```python
from build123d import *

# Parameters (mm, degrees)
EXTRUDE_1_DEPTH     = 1.5
HOLE_WIZARD_M4_1_D  = 4.2
HOLE_WIZARD_M8_1_D  = 8.25
SKETCH_8_R          = 3.5
CUT_EXTRUDE_1_DEPTH = 144.323608762
SKETCH_9_R          = 3.5
CUT_EXTRUDE_2_DEPTH = 144.323608762


with BuildPart() as part:
    # 草圖1 → 填料-伸長1 (new body)
    with BuildSketch(Plane.XY):
        with BuildLine():
            Line((9.519190028, -18.946187519), (9.519190028, -5.659090909))
            ThreePointArc((9.519190028, -5.659090909), (9.226296809, -4.951984128), (8.519190028, -4.659090909))
            Line((8.519190028, -4.659090909), (-70.48081017, -4.659090909))
            ThreePointArc((-70.48081017, -4.659090909), (-71.187916951, -4.951984128), (-71.48081017, -5.659090909))
            Line((-71.48081017, -5.659090909), (-71.48081017, -18.946187519))
            ThreePointArc((-71.48081017, -18.946187519), (-73.531062702, -23.895934988), (-78.48081017, -25.946187519))
            Line((-78.48081017, -25.946187519), (-84.980810071, -25.946187519))
            ThreePointArc((-84.980810071, -25.946187519), (-85.687916853, -26.239080738), (-85.980810071, -26.946187519))
            Line((-85.980810071, -26.946187519), (-85.980810071, -92.341911374))
            ThreePointArc((-85.980810071, -92.341911374), (-85.688840793, -93.048093006), (-84.983425077, -93.341907955))
            Line((-84.983425077, -93.341907955), (-78.583599692, -93.358643592))
            ThreePointArc((-78.583599692, -93.358643592), (-73.586751521, -95.475153852), (-71.603919064, -100.526538095))
            Line((-71.603919064, -100.526538095), (-71.918462387, -113.635102561))
            ThreePointArc((-71.918462387, -113.635102561), (-71.634287831, -114.357665047), (-70.918750149, -114.659090909))
            Line((-70.918750149, -114.659090909), (8.519190028, -114.659090909))
            ThreePointArc((8.519190028, -114.659090909), (9.226296809, -114.36619769), (9.519190028, -113.659090909))
            Line((9.519190028, -113.659090909), (9.519190028, -100.371994299))
            ThreePointArc((9.519190028, -100.371994299), (11.569442559, -95.422246831), (16.519190028, -93.371994299))
            Line((16.519190028, -93.371994299), (23.019189929, -93.371994299))
            ThreePointArc((23.019189929, -93.371994299), (23.72629671, -93.07910108), (24.019189929, -92.371994299))
            Line((24.019189929, -92.371994299), (24.019189929, -26.946187519))
            ThreePointArc((24.019189929, -26.946187519), (23.72629671, -26.239080738), (23.019189929, -25.946187519))
            Line((23.019189929, -25.946187519), (16.519190028, -25.946187519))
            ThreePointArc((16.519190028, -25.946187519), (11.569442559, -23.895934988), (9.519190028, -18.946187519))
        make_face()
    extrude(amount=EXTRUDE_1_DEPTH)

    # M4 螺旋的螺孔鑽1 (through all)
    with Locations(Plane(origin=(0, 0, 0), x_dir=(-1, 0, 0), z_dir=(0, 0, -1))):
        with Locations((79.980810071, -87.644049447), (-18.019189929, -87.644049447), (-18.019189929, -31.644049447), (79.980810071, -31.644049447)):
            Hole(HOLE_WIZARD_M4_1_D / 2)

    # M8 螺旋的螺孔鑽1 (through all)
    with Locations(Plane.XY.offset(1.5)):
        with Locations((-55.980810071, -89.659090909), (-25.980810071, -89.659090909)):
            Hole(HOLE_WIZARD_M8_1_D / 2)

    # 草圖8 → 除料-伸長1 (cut, through all)
    with BuildSketch(Plane.XY.offset(1.5)):
        with Locations((4.019190028, -101.159090909)):
            Circle(SKETCH_8_R)
    extrude(amount=-CUT_EXTRUDE_1_DEPTH, mode=Mode.SUBTRACT)

    # 草圖9 → 除料-伸長2 (cut, through all)
    with BuildSketch(Plane.XY.offset(1.5)):
        with Locations((-0.480809972, -13.659090909)):
            Circle(SKETCH_9_R)
        with Locations((-20.480809972, -13.659090909)):
            Circle(SKETCH_9_R)
    extrude(amount=-CUT_EXTRUDE_2_DEPTH, mode=Mode.SUBTRACT)


solid = part.part
```
Model file for the job. Use its own axes, mm. A direction names the side the tool comes from. Coordinates: 2 decimals unless noted, no trailing zeros. Order: outer loops, then holes, each group sorted by start corner. A loop starts at its lowest first (then second) coordinate and runs counter-clockwise, first axis right, second up. Notation, with made-up numbers: (-9.5, -29.5) -> (0.5, -29.5) arc R31 cw to (0.5, -1.5) -> close; hole circle Ø7 at (55.5, -8.5). An arc over 180 degrees is marked (long way). Answer as a JSON object with one key per item and string values. Group by question number.
1) Drill centre lines: L1, parallel to Y at x = -79.5, z = 1.25; L2, parallel to X at y = -87.5, z = 0.6; L3, parallel to Y at x = 16.5, z = 0.8. Where is each one in solid material? Low to high.
2) Pull direction X, two halves, no side cores. Call faces 3 (the face through (11.515, -95.477, 0.74)), 4 (the face through (-77.98, -31.01, 0.76)), 5 (the face through (-32, -59, 0)): +X half, -X half, draft (parallel to the pull), parting line (faces both ways), or undercut.
3) Cut at B-B, the plane x = 12. Write the cut outline in (y, z), then the cut area to 3 significant figures.
4) Which spindle directions (+Z, -Z, +X, -X, +Y, -Y) get a long thin tool onto all of the face, cutting with end or side? Do faces 1 (the face through (-73.64, -95.42, 0.74)), 2 (the face through (-25.44, -85.57, 0.74)). Say none if no direction does.
5) Flat gauge pins, fed straight in: pin 1 (6.5 mm diameter, centred on x = -20.48, y = -13.66, fed in from +Z); pin 2 (0.8 mm diameter, centred on y = -13.5, z = 1, fed in from +X); pin 3 (0.8 mm diameter, centred on x = 21.5, z = 1, fed in from +Y). Where does each tip first touch, or does it go through?
6) Cut at A-A, the plane z = 0.55. Count the separate pieces of the cut face and the enclosed holes in it, then the cut area to 3 significant figures.
Check values:
{
 "1": {"L1": "y = -93.36 to -89.69, -85.6 to -33.69, -29.6 to -25.95", "L2": "x = -85.98 to -82.08, -77.89 to -59.5, -52.47 to -29.5, -22.47 to 15.92, 20.11 to 24.02", "L3": "y = -93.37 to -89.09, -86.19 to -33.09, -30.19 to -25.95"},
 "2": {"face 3": "+X half", "face 4": "undercut", "face 5": "draft"},
 "3": {"outline": "(-95.03, 0) -> (-24.29, 0) -> (-24.29, 1.5) -> (-95.03, 1.5) -> close", "area": "106 mm²"},
 "4": {"face 1": "+Z, -Z, -X", "face 2": "+Z, -Z"},
 "5": {"pin 1": "passes through", "pin 2": "stops at x = 9.52", "pin 3": "stops at y = -25.95"},
 "6": {"separate pieces": "1", "enclosed holes": "9", "area": "10,600 mm²"}
}
